from build123d import *

# Parameters (mm, degrees)
SKETCH1_W           = 84.5
SKETCH1_H           = 61.7
BOSS_EXTRUDE1_DEPTH = 1.7
SKETCH2_W           = 8
SKETCH2_H           = 30.1
BOSS_EXTRUDE2_DEPTH = 10
BOSS_EXTRUDE2_TAPER = 11
SKETCH3_R           = 5
BOSS_EXTRUDE3_DEPTH = 11
SKETCH4_R           = 5
BOSS_EXTRUDE4_DEPTH = 11
SKETCH5_W           = 6
SKETCH5_H           = 12.8
BOSS_EXTRUDE5_DEPTH = 10.5
SKETCH6_R           = 1.5
CUT_EXTRUDE1_DEPTH  = 10
SKETCH7_R           = 1.5
CUT_EXTRUDE2_DEPTH  = 10
SKETCH8_R           = 1.5
CUT_EXTRUDE3_DEPTH  = 10
SKETCH9_R           = 1.5
CUT_EXTRUDE4_DEPTH  = 10


with BuildPart() as part:
    # Sketch1 → Boss-Extrude1 (new body)
    with BuildSketch(Plane.XY):
        with Locations((11.152950311, 11.889984472)):
            Rectangle(SKETCH1_W, SKETCH1_H)
    extrude(amount=BOSS_EXTRUDE1_DEPTH)

    # Sketch2 → Boss-Extrude2 (add)
    with BuildSketch(Plane.XY.offset(1.7)):
        with Locations((47.002950311, 12.089984472)):
            Rectangle(SKETCH2_W, SKETCH2_H)
    extrude(amount=BOSS_EXTRUDE2_DEPTH, taper=BOSS_EXTRUDE2_TAPER)

    # Sketch3 → Boss-Extrude3 (add)
    with BuildSketch(Plane.XY.offset(1.7)):
        with Locations((19.402950311, 11.889984472)):
            Circle(SKETCH3_R)
    extrude(amount=BOSS_EXTRUDE3_DEPTH)

    # Sketch4 → Boss-Extrude4 (add)
    with BuildSketch(Plane.XY.offset(1.7)):
        with Locations((34.702950311, 12.039984472)):
            Circle(SKETCH4_R)
    extrude(amount=BOSS_EXTRUDE4_DEPTH)

    # Sketch5 → Boss-Extrude5 (add)
    with BuildSketch(Plane.XY.offset(1.7)):
        with Locations((-27.097049689, 12.339984472)):
            Rectangle(SKETCH5_W, SKETCH5_H)
    extrude(amount=BOSS_EXTRUDE5_DEPTH)

    # Sketch6 → Cut-Extrude1 (cut)
    with BuildSketch(Plane.XY.offset(1.7)):
        with Locations((-28.097049689, -15.960015528)):
            Circle(SKETCH6_R)
    extrude(amount=-CUT_EXTRUDE1_DEPTH, mode=Mode.SUBTRACT)

    # Sketch7 → Cut-Extrude2 (cut)
    with BuildSketch(Plane.XY.offset(1.7)):
        with Locations((-28.097049689, 39.739984472)):
            Circle(SKETCH7_R)
    extrude(amount=-CUT_EXTRUDE2_DEPTH, mode=Mode.SUBTRACT)

    # Sketch8 → Cut-Extrude3 (cut)
    with BuildSketch(Plane.XY.offset(1.7)):
        with Locations((50.402950311, -15.960015528)):
            Circle(SKETCH8_R)
    extrude(amount=-CUT_EXTRUDE3_DEPTH, mode=Mode.SUBTRACT)

    # Sketch9 → Cut-Extrude4 (cut)
    with BuildSketch(Plane.XY.offset(1.7)):
        with Locations((50.402950311, 39.739984472)):
            Circle(SKETCH9_R)
    extrude(amount=-CUT_EXTRUDE4_DEPTH, mode=Mode.SUBTRACT)


solid = part.part
The listing builds one solid part. Answer for the finished solid, in the listing's coordinates (mm). A direction names the side the tool comes from. Give positions to 0.01 mm unless a question says otherwise; leave off trailing zeros. Loops run counter-clockwise (first coordinate to the right, second up) from the corner with the lowest first, then second, coordinate; pieces in that order, holes last. Notation, with made-up numbers: (27.5, -4.75) - (65.5, -4.75) arc R19 cw to (65.5, 2.25) - close; hole circle Ø1 at (19.25, -24). An arc over 180 degrees is marked (long way). Write each question's results on one line, items separated by ' | '.
1. Consider probe 1 along X at (y, z) = (15.5, 6.5); probe 2 along Z at (x, y) = (22.5, -4.5); probe 3 along X at (y, z) = (12, 3.75). Determine where each line is inside the solid, lowest interval first. Write a range as from..to.
Resolved:
probe 1: x = -30.1..-24.1, 15.94..22.86, 31.09..38.31, 43.94..50.07 | probe 2: z = 0..1.7 | probe 3: x = -30.1..-24.1, 14.4..24.4, 29.7..39.7, 43.4..50.6
2. Which of the six approach directions +Z, -Z, +X, -X, +Y, -Y give full straight-line access (tool end or side, diameter ignored) to faces 1 (the face through (47, 12, 11.7)), 2 (the face through (15.72, 15.27, 7.12)), 3 (the face through (-27, 18.74, 7)), 4 (the face through (-27, 5.94, 7))?
Resolved:
face 1: +Z, +X, +Y, -Y | face 2: +Z | face 3: +Z, -X, +Y | face 4: +Z, -X, -Y
3. Find section C-C, the plane x = 32.5. Write down the section's boundary in (y, z).
Resolved:
outline: (-18.96, 0) - (42.74, 0) - (42.74, 1.7) - (16.53, 1.7) - (16.53, 12.7) - (7.55, 12.7) - (7.55, 1.7) - (-18.96, 1.7) - close
4. For a pull along Y with two mould halves and no side action, classify faces 5 (the face through (11, 42.74, 1)), 6 (the face through (-28.422, 38.276, 0.862)), 7 (the face through (11, 12, 0)) as +Y half, -Y half, draft (parallel to the pull), parting line (faces both ways), or undercut.
Resolved:
face 5: +Y half | face 6: undercut | face 7: draft
5. Find section A-A, the plane z = 5.75. Write down the section's boundary in (x, y), then the cut area to 3 significant figures.
Resolved:
outline: (-30.1, 5.94) - (-24.1, 5.94) - (-24.1, 18.74) - (-30.1, 18.74) - close; circle Ø10 at (19.4, 11.89); circle Ø10 at (34.7, 12.04); (43.79, -2.17) - (50.22, -2.17) - (50.22, 26.35) - (43.79, 26.35) - close | area: 417 mm^2
6. Find section D-D, the plane z = 9.75. Write down the section's boundary in (x, y), then the cut area to 3 significant figures.
Resolved:
outline: (-30.1, 5.94) - (-24.1, 5.94) - (-24.1, 18.74) - (-30.1, 18.74) - close; circle Ø10 at (19.4, 11.89); circle Ø10 at (34.7, 12.04); (44.57, -1.4) - (49.44, -1.4) - (49.44, 25.58) - (44.57, 25.58) - close | area: 365 mm^2
7. Find section B-B, the plane y = 24. Write down the section's boundary in (x, z).
Resolved:
outline: (-31.1, 0) - (53.4, 0) - (53.4, 1.7) - (51, 1.7) - (49.06, 11.7) - (44.95, 11.7) - (43, 1.7) - (-31.1, 1.7) - close
8. Flat-ended cylindrical pins translate along their axes: P1, Ø6.5, axis at x = -27, y = 15, coming from the +Z side; P2, Ø1, axis at x = 37.5, z = 7.5, coming from the -Y side; P3, Ø5, axis at x = 22.5, z = 8, coming from the +Y side. Find the tip coordinate at first contact, or state that the pin passes through.
Resolved:
P1: stops at z = 12.2 | P2: stops at y = 7.6 | P3: stops at y = 16.85
